```python
from build123d import *

# Parameters (mm, degrees)
PAD_DEPTH            = 18
POCKET_DEPTH         = 52.501
POCKET_DEPTH_BACK    = -52.501
POCKET001_DEPTH      = 52.501
POCKET001_DEPTH_BACK = -52.501
SKETCH003_W          = 57.660323
SKETCH003_H          = 78
PAD001_DEPTH         = 7
FILLET_R             = 8
FILLET001_R          = 5


with BuildPart() as part:
    # Sketch → Pad (new body)
    with BuildSketch(Plane.XY):
        Polygon((-97.028, -52.5), (-97.028, 52.5), (0, 45), (0, -45), align=None)
    extrude(amount=PAD_DEPTH)

    # Sketch001 → Pocket (cut, two sides)
    with BuildSketch(Plane(origin=(-97.028, 0, 0), x_dir=(1, 0, 0), z_dir=(0, -1, 0))) as pocket_sk:
        Polygon((0, 18), (3, 0), (0, 0), align=None)
    extrude(amount=-POCKET_DEPTH, mode=Mode.SUBTRACT)
    extrude(pocket_sk.sketch, amount=-POCKET_DEPTH_BACK, mode=Mode.SUBTRACT)

    # Sketch002 → Pocket001 (cut, two sides)
    with BuildSketch(Plane.XZ) as pocket001_sk:
        Polygon((-97.028, 18), (0, 14), (0, 18), align=None)
    extrude(amount=-POCKET001_DEPTH, mode=Mode.SUBTRACT)
    extrude(pocket001_sk.sketch, amount=-POCKET001_DEPTH_BACK, mode=Mode.SUBTRACT)

    # Sketch003 → Pad001 (join)
    with BuildSketch(Plane.XY):
        with Locations((-62.907697, 0)):
            Rectangle(SKETCH003_W, SKETCH003_H)
    extrude(amount=-PAD001_DEPTH)

    # Fillet
    fillet_edges = [part.edges().sort_by_distance(p)[0] for p in [
        (0, 0, 14),
    ]]
    fillet(fillet_edges, radius=FILLET_R)

    # Fillet001
    fillet001_edges = [part.edges().sort_by_distance(p)[0] for p in [
        (-52.349239, -49.046454, 16.158109),
        (-52.349239, 49.046454, 16.158109),
    ]]
    fillet(fillet001_edges, radius=FILLET001_R)


solid = part.part
```
Here's how the part is built. I have some questions about the finished solid (model axes, mm). A direction names the side the tool comes from. Coordinates: 2 decimals unless noted, no trailing zeros. Order: outer loops, then holes, each group sorted by start corner. A loop starts at its lowest first (then second) coordinate and runs counter-clockwise, first axis right, second up.
Item 1: If we section it at A-A, the plane y = 34: List the corners of the cut face in (x, z) for me.
Response values:
outline: (-97.03, 18) - (-94.03, 0) - (-91.74, 0) - (-91.74, -7) - (-34.08, -7) - (-34.08, 0) - (0, 0) - (0, 6.32) arc R8 ccw to (-7.67, 14.32) - close
Item 2: Which directions (+Z, -Z, +X, -X, +Y, -Y) give clear straight access to the entire face, cutting with the end or side of a thin tool? Please do faces 1 (the face through (-63, -39, -3)), 2 (the face through (-34.078, -1, -3)), 3 (the face through (-63, 39, -3)).
Response values:
face 1: -Z, +X, -X, -Y
face 2: -Z, +X, +Y, -Y
face 3: -Z, +X, -X, +Y
Item 3: If we section it at B-B, the plane z = -2.5: List the corners of the cut face in (x, y) for me.
Response values:
outline: (-91.74, -39) - (-34.08, -39) - (-34.08, 39) - (-91.74, 39) - close
Item 4: I'm going to push flat-ended pins straight in: pin 1 Ø3.5 at (x, z) = (-54, -3) entering from +Y; pin 2 Ø5 at (x, z) = (-84, -2) entering from -Y; pin 3 Ø5.5 at (x, z) = (-68.5, -5) entering from -Y. Where does each tip first touch, or does it pass through?
Response values:
pin 1: stops at y = 39
pin 2: stops at y = -51.61
pin 3: stops at y = -39
Item 5: I need wall thicknesses on probe 1 along Y at (x, z) = (-39, -5.5); probe 2 along Y at (x, z) = (-32, 10.25); probe 3 along Z at (x, y) = (-50.5, 35.5). Which ranges of each line are inside material? Lowest first, please.
Response values:
probe 1: y = -39 to 39
probe 2: y = -47.47 to 47.47
probe 3: z = -7 to 16.08
